Geometry check sheet. Reference: the model listing, model coordinates, mm. Face numbers are marked on the shaded views. A direction names the side the tool comes from. Give positions to 0.01 mm unless a question says otherwise; leave off trailing zeros. Write each loop counter-clockwise with the first axis right and the second up, starting at its lowest first coordinate (ties: lowest second). Pieces come first, ordered by that corner, then holes. Notation, with made-up numbers: (-31, 0) -> (-26, 0) arc R32 cw to (-26, 38) -> close; hole circle Ø3 at (2, -26). An arc over 180 degrees is marked (long way). Write item = value, one per line. Start each with the question number.
1. Cross-section at A-A, the plane x = 1.5. Record the cut outline in (y, z), plus the area to 3 significant figures.
2. Mould release check, pull along Y, two halves, no side actions. Record for the marked faces 3, 4, 5 and 6: pulls with the +Y half, pulls with the -Y half, needs draft (parallel to the pull), parting line crosses it, or undercut.
3. Thickness scan on line 1 along Y through (x, z) = (-5, 2.25); line 2 along X through (y, z) = (1, 2.4); line 3 along Y through (x, z) = (-2, 2.9). Record the ranges inside material, lowest first.
4. Cross-section at C-C, the plane y = -13. Record the cut outline in (x, z).
5. Cross-section at B-B, the plane z = 0.6. Record the cut outline in (x, y), plus the area to 3 significant figures.
6. Set-up check for the marked faces 1 and 2: record each of +Z, -Z, +X, -X, +Y, -Y from which the full face is reachable in a straight line by a thin tool's end or side.
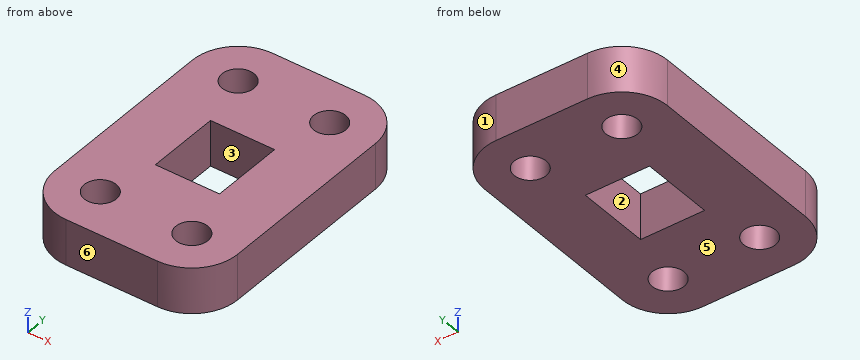
```python
from build123d import *

# Parameters (mm, degrees)
F0_R     = 1.75
F0_W     = 7
F0_H     = 8
F1_DEPTH = 5


with BuildPart() as f1:
    # F0 (on Top) → F1 (new body)
    with BuildSketch(Plane.XY):
        with BuildLine():
            ThreePointArc((-5, 15), (-8.535534, 13.535534), (-10, 10))
            Line((-10, 10), (-10, -10))
            ThreePointArc((-10, -10), (-8.535534, -13.535534), (-5, -15))
            Line((-5, -15), (5, -15))
            ThreePointArc((5, -15), (8.535534, -13.535534), (10, -10))
            Line((10, -10), (10, 10))
            ThreePointArc((10, 10), (8.535534, 13.535534), (5, 15))
            Line((5, 15), (-5, 15))
        make_face()
        with Locations((-5, -10)):
            Circle(F0_R, mode=Mode.SUBTRACT)
        with Locations((5, -10)):
            Circle(F0_R, mode=Mode.SUBTRACT)
        with Locations((-5, 10)):
            Circle(F0_R, mode=Mode.SUBTRACT)
        Rectangle(F0_W, F0_H, mode=Mode.SUBTRACT)
        with Locations((5, 10)):
            Circle(F0_R, mode=Mode.SUBTRACT)
    extrude(amount=F1_DEPTH)


solid = f1.part
```
Answers:
q1.outline = (-15, 0) -> (-4, 0) -> (-4, 5) -> (-15, 5) -> close; (4, 0) -> (15, 0) -> (15, 5) -> (4, 5) -> close
q1.area = 110 mm^2
q2.face_3 = undercut
q2.face_4 = pulls with the +Y half
q2.face_5 = needs draft
q2.face_6 = pulls with the -Y half
q3.line_1 = -15 to -11.75, -8.25 to 8.25, 11.75 to 15
q3.line_2 = -10 to -3.5, 3.5 to 10
q3.line_3 = -15 to -4, 4 to 15
q4.outline = (-9, 0) -> (9, 0) -> (9, 5) -> (-9, 5) -> close
q5.outline = (-10, -10) arc R5 ccw to (-5, -15) -> (5, -15) arc R5 ccw to (10, -10) -> (10, 10) arc R5 ccw to (5, 15) -> (-5, 15) arc R5 ccw to (-10, 10) -> close; hole circle Ø3.5 at (-5, -10); hole circle Ø3.5 at (-5, 10); hole (-3.5, -4) -> (3.5, -4) -> (3.5, 4) -> (-3.5, 4) -> close; hole circle Ø3.5 at (5, -10); hole circle Ø3.5 at (5, 10)
q5.area = 484 mm^2
q6.face_1 = +Z, -Z, +X, +Y
q6.face_2 = +Z, -Z
